```python
from build123d import *

# Parameters (mm, degrees)
SKETCH1_R            = 2.286
MAIN_BODY_DEPTH      = 1.5875
SKETCH13_R           = 6.28142
SKETCH13_R_2         = 2.286
BOSS_EXTRUDE9_DEPTH  = 6.35
CUT_EXTRUDE3_REACH   = 3.587
SKETCH5_R            = 1.5875
SKETCH5_R_2          = 2.286
SKETCH14_W           = 7.62
SKETCH14_H           = 6.35
BOSS_EXTRUDE10_DEPTH = 1.5875


with BuildPart() as part:
    # Sketch1 → Main Body (new body)
    with BuildSketch(Plane(origin=(0, 0, 0), x_dir=(1, 0, 0), z_dir=(0, 1, 0))):
        Polygon((-25.4, 86.995), (-63.43142, 86.995), (-63.43142, 60.96), (-78.74, 60.96), (-78.74, 25.4), (-71.12, 25.4), (-71.12, -25.4), (-78.74, -25.4), (-78.74, -60.96), (-63.43142, -60.96), (-63.43142, -86.995), (-25.4, -86.995), (-25.4, -79.375), (25.4, -79.375), (25.4, -86.995), (63.43142, -86.995), (63.43142, -60.96), (78.74, -60.96), (78.74, -25.4), (71.12, -25.4), (71.12, 25.4), (78.74, 25.4), (78.74, 60.96), (63.43142, 60.96), (63.43142, 86.995), (25.4, 86.995), (25.4, 79.375), (-25.4, 79.375), align=None)
        with Locations((-57.15, 76.2)):
            Circle(SKETCH1_R, mode=Mode.SUBTRACT)
        with Locations((57.15, 76.2)):
            Circle(SKETCH1_R, mode=Mode.SUBTRACT)
        with Locations((57.15, -76.2)):
            Circle(SKETCH1_R, mode=Mode.SUBTRACT)
        with Locations((-57.15, -76.2)):
            Circle(SKETCH1_R, mode=Mode.SUBTRACT)
    extrude(amount=MAIN_BODY_DEPTH)

    # Sketch13 → Boss-Extrude9 (add)
    with BuildSketch(Plane(origin=(0, 1.5875, 0), x_dir=(1, 0, 0), z_dir=(0, 1, 0))):
        with Locations((-57.15, 76.2)):
            Circle(SKETCH13_R)
        with Locations((-57.15, 76.2)):
            Circle(SKETCH13_R_2, mode=Mode.SUBTRACT)
        with Locations((-57.15, -76.2)):
            Circle(SKETCH13_R)
        with Locations((-57.15, -76.2)):
            Circle(SKETCH13_R_2, mode=Mode.SUBTRACT)
        with Locations((57.15, -76.2)):
            Circle(SKETCH13_R)
        with Locations((57.15, -76.2)):
            Circle(SKETCH13_R_2, mode=Mode.SUBTRACT)
        with Locations((57.15, 76.2)):
            Circle(SKETCH13_R)
        with Locations((57.15, 76.2)):
            Circle(SKETCH13_R_2, mode=Mode.SUBTRACT)
    extrude(amount=BOSS_EXTRUDE9_DEPTH)

    # Sketch5 → Cut-Extrude3 (cut, up to next)
    with BuildSketch(Plane(origin=(0, 1.5875, 0), x_dir=(1, 0, 0), z_dir=(0, 1, 0)), mode=Mode.PRIVATE) as cut_extrude3_sk1:
        with Locations((18.796, 30.734)):
            Circle(SKETCH5_R)
    cut_extrude3_tool1 = extrude(cut_extrude3_sk1.sketch, amount=-CUT_EXTRUDE3_REACH, mode=Mode.PRIVATE) & part.part
    add(cut_extrude3_tool1.solids().sort_by_distance((18.796, 1.5875, -30.734))[0], mode=Mode.SUBTRACT)
    # Sketch5 → Cut-Extrude3 (cut, up to next)
    with BuildSketch(Plane(origin=(0, 1.5875, 0), x_dir=(1, 0, 0), z_dir=(0, 1, 0)), mode=Mode.PRIVATE) as cut_extrude3_sk2:
        with Locations((73.406, 30.734)):
            Circle(SKETCH5_R)
    cut_extrude3_tool2 = extrude(cut_extrude3_sk2.sketch, amount=-CUT_EXTRUDE3_REACH, mode=Mode.PRIVATE) & part.part
    add(cut_extrude3_tool2.solids().sort_by_distance((73.406, 1.5875, -30.734))[0], mode=Mode.SUBTRACT)
    # Sketch5 → Cut-Extrude3 (cut, up to next)
    with BuildSketch(Plane(origin=(0, 1.5875, 0), x_dir=(1, 0, 0), z_dir=(0, 1, 0)), mode=Mode.PRIVATE) as cut_extrude3_sk3:
        with Locations((73.406, -30.988)):
            Circle(SKETCH5_R)
    cut_extrude3_tool3 = extrude(cut_extrude3_sk3.sketch, amount=-CUT_EXTRUDE3_REACH, mode=Mode.PRIVATE) & part.part
    add(cut_extrude3_tool3.solids().sort_by_distance((73.406, 1.5875, 30.988))[0], mode=Mode.SUBTRACT)
    # Sketch5 → Cut-Extrude3 (cut, up to next)
    with BuildSketch(Plane(origin=(0, 1.5875, 0), x_dir=(1, 0, 0), z_dir=(0, 1, 0)), mode=Mode.PRIVATE) as cut_extrude3_sk4:
        with Locations((18.796, -30.988)):
            Circle(SKETCH5_R)
    cut_extrude3_tool4 = extrude(cut_extrude3_sk4.sketch, amount=-CUT_EXTRUDE3_REACH, mode=Mode.PRIVATE) & part.part
    add(cut_extrude3_tool4.solids().sort_by_distance((18.796, 1.5875, 30.988))[0], mode=Mode.SUBTRACT)
    # Sketch5 → Cut-Extrude3 (cut, up to next)
    with BuildSketch(Plane(origin=(0, 1.5875, 0), x_dir=(1, 0, 0), z_dir=(0, 1, 0)), mode=Mode.PRIVATE) as cut_extrude3_sk5:
        with Locations((-28.575, 64.77)):
            Circle(SKETCH5_R)
    cut_extrude3_tool5 = extrude(cut_extrude3_sk5.sketch, amount=-CUT_EXTRUDE3_REACH, mode=Mode.PRIVATE) & part.part
    add(cut_extrude3_tool5.solids().sort_by_distance((-28.575, 1.5875, -64.77))[0], mode=Mode.SUBTRACT)
    # Sketch5 → Cut-Extrude3 (cut, up to next)
    with BuildSketch(Plane(origin=(0, 1.5875, 0), x_dir=(1, 0, 0), z_dir=(0, 1, 0)), mode=Mode.PRIVATE) as cut_extrude3_sk6:
        with Locations((45.085, 64.77)):
            Circle(SKETCH5_R)
    cut_extrude3_tool6 = extrude(cut_extrude3_sk6.sketch, amount=-CUT_EXTRUDE3_REACH, mode=Mode.PRIVATE) & part.part
    add(cut_extrude3_tool6.solids().sort_by_distance((45.085, 1.5875, -64.77))[0], mode=Mode.SUBTRACT)
    # Sketch5 → Cut-Extrude3 (cut, up to next)
    with BuildSketch(Plane(origin=(0, 1.5875, 0), x_dir=(1, 0, 0), z_dir=(0, 1, 0)), mode=Mode.PRIVATE) as cut_extrude3_sk7:
        with Locations((-66.04, 28.575)):
            Circle(SKETCH5_R)
    cut_extrude3_tool7 = extrude(cut_extrude3_sk7.sketch, amount=-CUT_EXTRUDE3_REACH, mode=Mode.PRIVATE) & part.part
    add(cut_extrude3_tool7.solids().sort_by_distance((-66.04, 1.5875, -28.575))[0], mode=Mode.SUBTRACT)
    # Sketch5 → Cut-Extrude3 (cut, up to next)
    with BuildSketch(Plane(origin=(0, 1.5875, 0), x_dir=(1, 0, 0), z_dir=(0, 1, 0)), mode=Mode.PRIVATE) as cut_extrude3_sk8:
        with Locations((-38.1, 64.135)):
            Circle(SKETCH5_R)
    cut_extrude3_tool8 = extrude(cut_extrude3_sk8.sketch, amount=-CUT_EXTRUDE3_REACH, mode=Mode.PRIVATE) & part.part
    add(cut_extrude3_tool8.solids().sort_by_distance((-38.1, 1.5875, -64.135))[0], mode=Mode.SUBTRACT)
    # Sketch5 → Cut-Extrude3 (cut, up to next)
    with BuildSketch(Plane(origin=(0, 1.5875, 0), x_dir=(1, 0, 0), z_dir=(0, 1, 0)), mode=Mode.PRIVATE) as cut_extrude3_sk9:
        with Locations((-38.1, 28.575)):
            Circle(SKETCH5_R)
    cut_extrude3_tool9 = extrude(cut_extrude3_sk9.sketch, amount=-CUT_EXTRUDE3_REACH, mode=Mode.PRIVATE) & part.part
    add(cut_extrude3_tool9.solids().sort_by_distance((-38.1, 1.5875, -28.575))[0], mode=Mode.SUBTRACT)
    # Sketch5 → Cut-Extrude3 (cut, up to next)
    with BuildSketch(Plane(origin=(0, 1.5875, 0), x_dir=(1, 0, 0), z_dir=(0, 1, 0)), mode=Mode.PRIVATE) as cut_extrude3_sk10:
        with Locations((-72.39, -54.61)):
            Circle(SKETCH5_R_2)
    cut_extrude3_tool10 = extrude(cut_extrude3_sk10.sketch, amount=-CUT_EXTRUDE3_REACH, mode=Mode.PRIVATE) & part.part
    add(cut_extrude3_tool10.solids().sort_by_distance((-72.39, 1.5875, 54.61))[0], mode=Mode.SUBTRACT)

    # Sketch14 → Boss-Extrude10 (add)
    with BuildSketch(Plane(origin=(0, 1.5875, 0), x_dir=(1, 0, 0), z_dir=(0, 1, 0))):
        with Locations((-74.93, -22.225)):
            Rectangle(SKETCH14_W, SKETCH14_H)
        with Locations((-74.93, 22.225)):
            Rectangle(SKETCH14_W, SKETCH14_H)
        with Locations((74.93, -22.225)):
            Rectangle(SKETCH14_W, SKETCH14_H)
        with Locations((74.93, 22.225)):
            Rectangle(SKETCH14_W, SKETCH14_H)
    extrude(amount=-BOSS_EXTRUDE10_DEPTH)


solid = part.part
```
CAD build for the part. Positions are in the model's coordinates, mm. A direction names the side the tool comes from. Round coordinates to 2 decimals unless told otherwise and drop trailing zeros. Write each loop counter-clockwise with the first axis right and the second up, starting at its lowest first coordinate (ties: lowest second). Pieces come first, ordered by that corner, then holes. Notation, with made-up numbers: (57.25, -10.5) - (63.25, -10.5) arc R13 cw to (63.25, 13.5) - close; hole circle Ø10 at (36.25, -32). An arc over 180 degrees is marked (long way). Return JSON: item names as keys, results as strings. Group by question number.
Item 1: Band-saw the part on B-B on y = 5.5. List the corners of the cut face in (x, z), plus the area to 3 significant figures.
Item 2: 3-axis set-ups, long thin cutter, end or side, ignore diameter. For faces 3 (the face through (-57, 7.938, 79)), 4 (the face through (-51.16, 4.72, 74.31)): which of +Z, -Z, +X, -X, +Y, -Y reach the whole face in a straight line?
Item 3: Mould opens along Z. For faces 1 (the face through (63.14, 4.72, -78.09)), 2 (the face through (57, 7.938, 79)) say: +Z half, -Z half, draft (parallel to the pull), parting line (faces both ways), or undercut.
Item 4: Band-saw the part on D-D on x = 34. List the corners of the cut face in (y, z) (1 decimal).
Item 5: Band-saw the part on A-A on x = -57.15. List the corners of the cut face in (y, z) (1 decimal).
Item 6: Probe probe 1 along Z at (x, y) = (-38.1, 0.65) (1 decimal); probe 2 along Z at (x, y) = (-57.15, 5.25); probe 3 along X at (y, z) = (0.85, -64.77). List the from-to ranges inside material, lowest first.
Item 7: Flat gauge pins, fed straight in: pin 1 Ø5 at (x, z) = (-28.575, -64.77) entering from +Y; pin 2 Ø5.5 at (x, z) = (57.15, 76.2) entering from -Y; pin 3 Ø2 at (y, z) = (5, -67) entering from -X; pin 4 Ø1.7 at (x, y) = (-72, 1) entering from +Z. Where does each tip first touch, or does it go through?
Item 8: Band-saw the part on C-C on z = 54.61. List the corners of the cut face in (x, y), plus the area to 3 significant figures.
Resolved:
{
 "1": {"outline": "circle Ø12.56 at (-57.15, -76.2); circle Ø12.56 at (-57.15, 76.2); circle Ø12.56 at (57.15, -76.2); circle Ø12.56 at (57.15, 76.2); hole circle Ø4.57 at (-57.15, -76.2); hole circle Ø4.57 at (-57.15, 76.2); hole circle Ø4.57 at (57.15, -76.2); hole circle Ø4.57 at (57.15, 76.2)", "area": "430 mm²"},
 "2": {"face 3": "+Z, -Z, +X, -X, +Y", "face 4": "+Y"},
 "3": {"face 1": "undercut", "face 2": "draft"},
 "4": {"outline": "(0, -87) - (1.6, -87) - (1.6, 87) - (0, 87) - close"},
 "5": {"outline": "(0, -87) - (1.6, -87) - (1.6, -82.5) - (7.9, -82.5) - (7.9, -78.5) - (0, -78.5) - close; (0, -73.9) - (7.9, -73.9) - (7.9, -69.9) - (1.6, -69.9) - (1.6, 69.9) - (7.9, 69.9) - (7.9, 73.9) - (0, 73.9) - close; (0, 78.5) - (7.9, 78.5) - (7.9, 82.5) - (1.6, 82.5) - (1.6, 87) - (0, 87) - close"},
 "6": {"probe 1": "z = -87 to -65.7, -62.5 to -30.2, -27 to 87", "probe 2": "z = -82.48 to -78.49, -73.91 to -69.92, 69.92 to 73.91, 78.49 to 82.48", "probe 3": "x = -63.43 to -39.55, -36.65 to -30.16, -26.99 to 43.5, 46.67 to 63.43"},
 "7": {"pin 1": "stops at y = 1.59", "pin 2": "stops at y = 0", "pin 3": "passes through", "pin 4": "stops at z = 60.96"},
 "8": {"outline": "(-78.74, 0) - (-74.68, 0) - (-74.68, 1.59) - (-78.74, 1.59) - close; (-70.1, 0) - (78.74, 0) - (78.74, 1.59) - (-70.1, 1.59) - close", "area": "243 mm²"}
}
